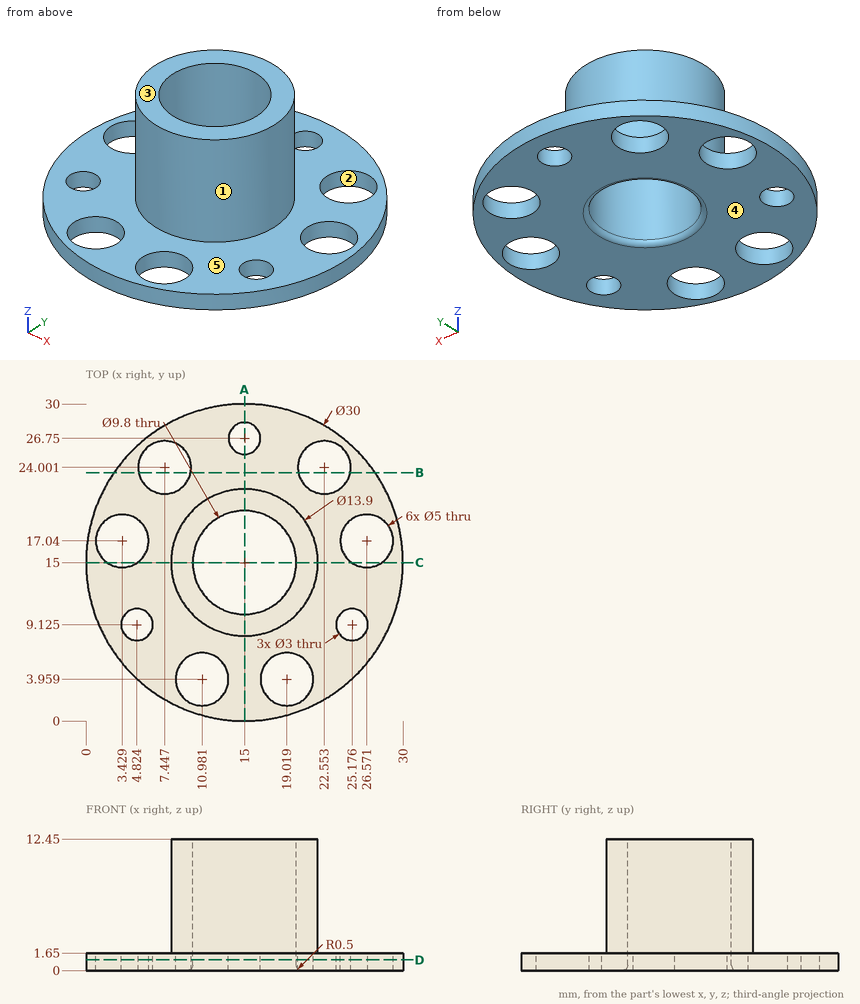
Here's the drawing with two shaded views (mm, measured from the low corner). I have some questions. A direction names the side the tool comes from. Round coordinates to 2 decimals unless told otherwise and drop trailing zeros. Write each loop counter-clockwise with the first axis right and the second up, starting at its lowest first coordinate (ties: lowest second). Pieces come first, ordered by that corner, then holes.
(1) Suppose I cut it at A-A on x = 15. Write out the boundary of the cut face in (y, z).
Findings below:
outline: (0, 0) - (9.6, 0) arc R0.5 ccw to (10.1, 0.5) - (10.1, 12.45) - (8.05, 12.45) - (8.05, 1.65) - (0, 1.65) - close; (19.9, 0.5) arc R0.5 ccw to (20.4, 0) - (25.25, 0) - (25.25, 1.65) - (21.95, 1.65) - (21.95, 12.45) - (19.9, 12.45) - close; (28.25, 0) - (30, 0) - (30, 1.65) - (28.25, 1.65) - close
(2) Suppose I cut it at B-B on y = 23.5. Write out the boundary of the cut face in (x, z).
Findings below:
outline: (2.64, 0) - (5, 0) - (5, 1.65) - (2.64, 1.65) - close; (9.9, 0) - (20.1, 0) - (20.1, 1.65) - (9.9, 1.65) - close; (25, 0) - (27.36, 0) - (27.36, 1.65) - (25, 1.65) - close
(3) If I drill on probe 1 along X at (y, z) = (23.75, 1) (1 decimal); probe 2 along Z at (x, y) = (26.5, 8.25), over which ranges is the centre line in solid material (lowest first)?
Findings below:
probe 1: x = 2.8 to 5, 9.9 to 20.1, 25 to 27.2
probe 2: z = 0 to 1.65
(4) For pin 1 (3 mm diameter, centred on x = 15.5, z = 8, fed in from +Y); pin 2 (6 mm diameter, centred on x = 3.43, y = 17.04, fed in from -Z); pin 3 (6 mm diameter, centred on x = 7.45, y = 24, fed in from +Z), each with a flat end and sliding along its axis, tell me the tip position at first contact or that it passes through.
Findings below:
pin 1: stops at y = 21.95
pin 2: stops at z = 0
pin 3: stops at z = 1.65
(5) Suppose I cut it at D-D on z = 1. State how many separate pieces and enclosed holes the cut face has.
Findings below:
separate pieces: 1
enclosed holes: 10
(6) Which directions (+Z, -Z, +X, -X, +Y, -Y) give clear straight access to the entire face, cutting with the end or side of a thin tool? Please do the marked faces 4 and 5.
Findings below:
face 4: -Z, +X, -X, +Y, -Y
face 5: +Z
(7) Thinking about a two-plate mould opening in X: for the marked faces 1, 2 and 3, which applies, +X half, -X half, draft (parallel to the pull), parting line (faces both ways), or undercut?
Findings below:
face 1: parting line
face 2: undercut
face 3: draft
(8) Suppose I cut it at C-C on y = 15. Write out the boundary of the cut face in (x, z).
Findings below:
outline: (0, 0) - (1.98, 0) - (1.98, 1.65) - (0, 1.65) - close; (4.87, 0) - (9.6, 0) arc R0.5 ccw to (10.1, 0.5) - (10.1, 12.45) - (8.05, 12.45) - (8.05, 1.65) - (4.87, 1.65) - close; (19.9, 0.5) arc R0.5 ccw to (20.4, 0) - (25.13, 0) - (25.13, 1.65) - (21.95, 1.65) - (21.95, 12.45) - (19.9, 12.45) - close; (28.02, 0) - (30, 0) - (30, 1.65) - (28.02, 1.65) - close
